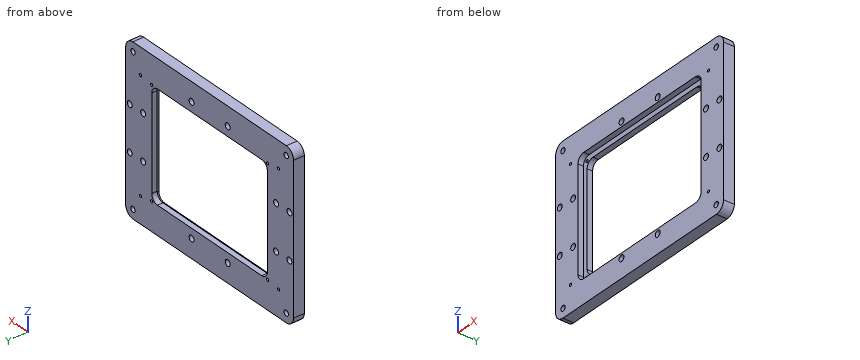
```python
from build123d import *

# Parameters (mm, degrees)
SKETCH_2_W               = 220
SKETCH_2_H               = 150
SKETCH_2_W_2             = 160
SKETCH_2_H_2             = 120
EXTRUDE_1_DEPTH          = 12
SKETCH_3_W               = 170.5
SKETCH_3_H               = 130.5
CUT_EXTRUDE_1_DEPTH      = 6
FILLET_1_R               = 8
FILLET_2_R               = 8
FILLET_3_R               = 8
CUT_EXTRUDE_2_DEPTH      = 134.270401815
CUT_EXTRUDE_2_DEPTH_BACK = 140.270401815
CUT_EXTRUDE_2_START      = 6
SKETCH_4_R               = 1.5
SKETCH_6_W               = 241.523327546
SKETCH_6_H               = 183.41982478
SKETCH_6_W_2             = 210.674446864
SKETCH_6_H_2             = 143.430858526
EXTRUDE_2_DEPTH          = 12
SKETCH_5_R               = 3.3655
CUT_EXTRUDE_3_DEPTH      = 22
SKETCH_7_R               = 3
CUT_EXTRUDE_4_DEPTH      = 22
FILLET_4_R               = 6
FILLET_5_R               = 6
FILLET_6_R               = 6
FILLET_7_R               = 6
SKETCH_14_W              = 180
SKETCH_14_H              = 7.031256172
SKETCH_14_R              = 2
EXTRUDE_3_DEPTH          = 12
SKETCH_14_W_2            = 130
SKETCH_14_H_2            = 7
EXTRUDE_3_2_DEPTH        = 12
EXTRUDE_3_3_DEPTH        = 12
EXTRUDE_3_4_DEPTH        = 12
SKETCH_15_W              = 460.716543434
SKETCH_15_H              = 403.643057854
SKETCH_15_W_2            = 232.32954725
SKETCH_15_H_2            = 183.087092282
CUT_EXTRUDE_8_DEPTH      = 105
FILLET_8_R               = 10


with BuildPart() as part:
    # Эскиз2 → Бобышка-Вытянуть1 (new body)
    with BuildSketch(Plane(origin=(0, 0, 0), x_dir=(1, 0, 0), z_dir=(0, 1, 0))):
        Rectangle(SKETCH_2_W, SKETCH_2_H)
        Rectangle(SKETCH_2_W_2, SKETCH_2_H_2, mode=Mode.SUBTRACT)
    extrude(amount=EXTRUDE_1_DEPTH)

    # Эскиз3 → Вырез-Вытянуть1 (cut)
    with BuildSketch(Plane.XZ):
        Rectangle(SKETCH_3_W, SKETCH_3_H)
    extrude(amount=-CUT_EXTRUDE_1_DEPTH, mode=Mode.SUBTRACT)

    # Скругление1
    fillet_1_edges = [part.edges().sort_by_distance(p)[0] for p in [
        (80, 9, 60),
    ]]
    fillet(fillet_1_edges, radius=FILLET_1_R)

    # Скругление2
    fillet_2_edges = [part.edges().sort_by_distance(p)[0] for p in [
        (85.25, 3, 65.25),
    ]]
    fillet(fillet_2_edges, radius=FILLET_2_R)

    # Скругление3
    fillet_3_edges = [part.edges().sort_by_distance(p)[0] for p in [
        (80, 9, -60),
        (-80, 9, -60),
        (-80, 9, 60),
        (85.25, 3, -65.25),
        (-85.25, 3, -65.25),
        (-85.25, 3, 65.25),
    ]]
    fillet(fillet_3_edges, radius=FILLET_3_R)

    # Эскиз4 → Вырез-Вытянуть2 (cut, two sides: drawn at the far end of the back side and taken through both)
    with BuildSketch(Plane.XZ.offset(-6).offset(CUT_EXTRUDE_2_START - CUT_EXTRUDE_2_DEPTH_BACK)):
        with Locations(Location((-80.15, 60.15, 0), (0, 0, 270))):
            Circle(SKETCH_4_R)
        with Locations(Location((-80.15, -60.15, 0), (0, 0, 270))):
            Circle(SKETCH_4_R)
        with Locations(Location((80.15, -60.15, 0), (0, 0, 270))):
            Circle(SKETCH_4_R)
        with Locations(Location((80.15, 60.15, 0), (0, 0, 270))):
            Circle(SKETCH_4_R)
        with Locations(Location((-95.5, 62.5, 0), (0, 0, 270))):
            Circle(SKETCH_4_R)
        with Locations(Location((-95.5, -62.5, 0), (0, 0, 270))):
            Circle(SKETCH_4_R)
        with Locations(Location((95.5, -62.5, 0), (0, 0, 270))):
            Circle(SKETCH_4_R)
        with Locations(Location((95.5, 62.5, 0), (0, 0, 270))):
            Circle(SKETCH_4_R)
    extrude(amount=CUT_EXTRUDE_2_DEPTH + CUT_EXTRUDE_2_DEPTH_BACK, mode=Mode.SUBTRACT)

    # Эскиз6 → Бобышка-Вытянуть2 (add)
    with BuildSketch(Plane.XZ):
        Rectangle(SKETCH_6_W, SKETCH_6_H)
        Rectangle(SKETCH_6_W_2, SKETCH_6_H_2, mode=Mode.SUBTRACT)
    extrude(amount=-EXTRUDE_2_DEPTH)

    # Эскиз5 → Вырез-Вытянуть3 (cut)
    with BuildSketch(Plane.XZ):
        with Locations(Location((-92.006407499, -25, 0), (0, 0, 270))):
            Circle(SKETCH_5_R)
        with Locations(Location((-110.497607499, -25, 0), (0, 0, 270))):
            Circle(SKETCH_5_R)
        with Locations(Location((-110.497607499, 25.000000038, 0), (0, 0, 270))):
            Circle(SKETCH_5_R)
        with Locations(Location((-92.006407499, 25.000000038, 0), (0, 0, 270))):
            Circle(SKETCH_5_R)
        with Locations(Location((92.006407499, 25.000000038, 0), (0, 0, 270))):
            Circle(SKETCH_5_R)
        with Locations(Location((110.497607499, 25.000000038, 0), (0, 0, 270))):
            Circle(SKETCH_5_R)
        with Locations(Location((110.497607499, -25, 0), (0, 0, 270))):
            Circle(SKETCH_5_R)
        with Locations(Location((92.006407499, -25, 0), (0, 0, 270))):
            Circle(SKETCH_5_R)
        with Locations(Location((25, 70.661122045, 0), (0, 0, 270))):
            Circle(SKETCH_5_R)
        with Locations(Location((-25.000000038, 70.661122045, 0), (0, 0, 270))):
            Circle(SKETCH_5_R)
        with Locations(Location((-25.000000038, -70.661122045, 0), (0, 0, 270))):
            Circle(SKETCH_5_R)
        with Locations(Location((25, -70.661122045, 0), (0, 0, 270))):
            Circle(SKETCH_5_R)
    extrude(amount=-CUT_EXTRUDE_3_DEPTH, mode=Mode.SUBTRACT)

    # Эскиз7 → Вырез-Вытянуть4 (cut)
    with BuildSketch(Plane.XZ):
        with Locations(Location((-106.020205838, -81.450824183, 0), (0, 0, 270))):
            Circle(SKETCH_7_R)
        with Locations(Location((-106.020205838, 81.450824183, 0), (0, 0, 270))):
            Circle(SKETCH_7_R)
        with Locations(Location((106.020205838, 81.450824183, 0), (0, 0, 270))):
            Circle(SKETCH_7_R)
        with Locations(Location((106.020205838, -81.450824183, 0), (0, 0, 270))):
            Circle(SKETCH_7_R)
    extrude(amount=-CUT_EXTRUDE_4_DEPTH, mode=Mode.SUBTRACT)

    # Скругление4
    fillet_4_edges = [part.edges().sort_by_distance(p)[0] for p in [
        (120.761663773, 6, 91.70991239),
    ]]
    fillet(fillet_4_edges, radius=FILLET_4_R)

    # Скругление5
    fillet_5_edges = [part.edges().sort_by_distance(p)[0] for p in [
        (120.761663773, 6, -91.70991239),
    ]]
    fillet(fillet_5_edges, radius=FILLET_5_R)

    # Скругление6
    fillet_6_edges = [part.edges().sort_by_distance(p)[0] for p in [
        (-120.761663773, 6, -91.70991239),
    ]]
    fillet(fillet_6_edges, radius=FILLET_6_R)

    # Скругление7
    fillet_7_edges = [part.edges().sort_by_distance(p)[0] for p in [
        (-120.761663773, 6, 91.70991239),
    ]]
    fillet(fillet_7_edges, radius=FILLET_7_R)


with BuildPart() as body_2:
    # Эскиз14 → Бобышка-Вытянуть3 (new body)
    with BuildSketch(Plane(origin=(0, 12, 0), x_dir=(1, 0, 0), z_dir=(0, 1, 0))):
        with Locations((1.41446019, 109.44602362)):
            Rectangle(SKETCH_14_W, SKETCH_14_H)
        with Locations(Location((-81.58561634, 109.413291168, 0), (0, 0, 270))):
            Circle(SKETCH_14_R, mode=Mode.SUBTRACT)
        with Locations(Location((1.41446019, 109.413291168, 0), (0, 0, 270))):
            Circle(SKETCH_14_R, mode=Mode.SUBTRACT)
        with Locations(Location((84.41453672, 109.413291168, 0), (0, 0, 270))):
            Circle(SKETCH_14_R, mode=Mode.SUBTRACT)
    extrude(amount=-EXTRUDE_3_DEPTH)


with BuildPart() as body_3:
    # Эскиз14 → Extrude 3 2 (new body)
    with BuildSketch(Plane(origin=(0, 12, 0), x_dir=(1, 0, 0), z_dir=(0, 1, 0))):
        with Locations((-6.451217143, 118.582116541)):
            Rectangle(SKETCH_14_W_2, SKETCH_14_H_2)
        with Locations(Location((51.548782857, 118.582116541, 0), (0, 0, 270))):
            Circle(SKETCH_14_R, mode=Mode.SUBTRACT)
        with Locations(Location((-6.451217143, 118.582116541, 0), (0, 0, 270))):
            Circle(SKETCH_14_R, mode=Mode.SUBTRACT)
        with Locations(Location((-64.451217143, 118.582116541, 0), (0, 0, 270))):
            Circle(SKETCH_14_R, mode=Mode.SUBTRACT)
    extrude(amount=-EXTRUDE_3_2_DEPTH)


with BuildPart() as body_4:
    # Эскиз14 → Extrude 3 3 (new body)
    with BuildSketch(Plane(origin=(0, 12, 0), x_dir=(1, 0, 0), z_dir=(0, 1, 0))):
        with Locations((1.538593971, 129.106977772)):
            Rectangle(SKETCH_14_W, SKETCH_14_H)
        with Locations(Location((-81.461482559, 129.07424532, 0), (0, 0, 270))):
            Circle(SKETCH_14_R, mode=Mode.SUBTRACT)
        with Locations(Location((1.538593971, 129.07424532, 0), (0, 0, 270))):
            Circle(SKETCH_14_R, mode=Mode.SUBTRACT)
        with Locations(Location((84.538670501, 129.07424532, 0), (0, 0, 270))):
            Circle(SKETCH_14_R, mode=Mode.SUBTRACT)
    extrude(amount=-EXTRUDE_3_3_DEPTH)


with BuildPart() as body_5:
    # Эскиз14 → Extrude 3 4 (new body)
    with BuildSketch(Plane(origin=(0, 12, 0), x_dir=(1, 0, 0), z_dir=(0, 1, 0))):
        with Locations((-6.327083362, 138.243070693)):
            Rectangle(SKETCH_14_W_2, SKETCH_14_H_2)
        with Locations(Location((51.672916638, 138.243070693, 0), (0, 0, 270))):
            Circle(SKETCH_14_R, mode=Mode.SUBTRACT)
        with Locations(Location((-6.327083362, 138.243070693, 0), (0, 0, 270))):
            Circle(SKETCH_14_R, mode=Mode.SUBTRACT)
        with Locations(Location((-64.327083362, 138.243070693, 0), (0, 0, 270))):
            Circle(SKETCH_14_R, mode=Mode.SUBTRACT)
    extrude(amount=-EXTRUDE_3_4_DEPTH)


with BuildPart() as cut_extrude_8_tool:
    # Эскиз15 → Вырез-Вытянуть8 (new body)
    with BuildSketch(Plane.XZ):
        Rectangle(SKETCH_15_W, SKETCH_15_H)
        Rectangle(SKETCH_15_W_2, SKETCH_15_H_2, mode=Mode.SUBTRACT)
    extrude(amount=-CUT_EXTRUDE_8_DEPTH)


with BuildPart() as part_1:
    add(part.part)

    # Вырез-Вытянуть8: cut by cut_extrude_8_tool
    add(cut_extrude_8_tool.part, mode=Mode.SUBTRACT)

    # Скругление8
    fillet_8_edges = [part_1.edges().sort_by_distance(p)[0] for p in [
        (116.164773625, 6, -91.543546141),
        (-116.164773625, 6, -91.543546141),
        (-116.164773625, 6, 91.543546141),
        (116.164773625, 6, 91.543546141),
    ]]
    fillet(fillet_8_edges, radius=FILLET_8_R)


with BuildPart() as body_2_1:
    add(body_2.part)

    # Вырез-Вытянуть8: cut by cut_extrude_8_tool
    add(cut_extrude_8_tool.part, mode=Mode.SUBTRACT)


with BuildPart() as body_3_1:
    add(body_3.part)

    # Вырез-Вытянуть8: cut by cut_extrude_8_tool
    add(cut_extrude_8_tool.part, mode=Mode.SUBTRACT)


with BuildPart() as body_4_1:
    add(body_4.part)

    # Вырез-Вытянуть8: cut by cut_extrude_8_tool
    add(cut_extrude_8_tool.part, mode=Mode.SUBTRACT)


with BuildPart() as body_5_1:
    add(body_5.part)

    # Вырез-Вытянуть8: cut by cut_extrude_8_tool
    add(cut_extrude_8_tool.part, mode=Mode.SUBTRACT)


solid = part_1.part
```
The listing builds one solid part. Answer for the finished solid, in the listing's coordinates (mm). Give positions to 0.01 mm unless a question says otherwise; leave off trailing zeros. Write each loop counter-clockwise with the first axis right and the second up, starting at its lowest first coordinate (ties: lowest second). Pieces come first, ordered by that corner, then holes. Notation, with made-up numbers: (64, 33) - (69, 33) arc R12 cw to (69, 51) - close; hole circle Ø9 at (6.25, 9). An arc over 180 degrees is marked (long way). Use one line per item in the form item = value. Start each with the question number.
1) Find section B-B on z = 25. Determine the outline of the cut face in (x, y), plus the area to 3 significant figures.
2) Find section C-C on z = 71. Determine the outline of the cut face in (x, y).
3) Find section D-D on y = 3.5. Count the separate pieces of the cut face and the enclosed holes in it, plus the area to 3 significant figures.
4) Find section A-A on x = 25. Determine the outline of the cut face in (y, z).
5) A flat-ended cylindrical pin translates along its axis: pin 1 Ø4 at (x, z) = (-92.01, -25) entering from -Y. Find the tip coordinate at first contact, or state that the pin passes through.
6) Consider line 1 along Z through (x, y) = (25.5, 3.75); line 2 along X through (y, z) = (8.7, -60.15); line 3 along Z through (x, y) = (-54, 11.25). Determine where each line is inside the solid, lowest interval first. Write a range as from..to.
Geometry results:
q1.outline = (-116.16, 0) - (-113.86, 0) - (-113.86, 12) - (-116.16, 12) - close; (-107.13, 0) - (-95.37, 0) - (-95.37, 12) - (-107.13, 12) - close; (-88.64, 0) - (-85.25, 0) - (-85.25, 6) - (-80, 6) - (-80, 12) - (-88.64, 12) - close; (80, 6) - (85.25, 6) - (85.25, 0) - (88.64, 0) - (88.64, 12) - (80, 12) - close; (95.37, 0) - (107.13, 0) - (107.13, 12) - (95.37, 12) - close; (113.86, 0) - (116.16, 0) - (116.16, 12) - (113.86, 12) - close
q1.area = 482 mm2
q2.outline = (-116.16, 0) - (-28.35, 0) - (-28.35, 12) - (-116.16, 12) - close; (-21.65, 0) - (21.65, 0) - (21.65, 12) - (-21.65, 12) - close; (28.35, 0) - (116.16, 0) - (116.16, 12) - (28.35, 12) - close
q3.separate_pieces = 1
q3.enclosed_holes = 21
q3.area = 19,700 mm2
q4.outline = (0, -91.54) - (12, -91.54) - (12, -74.03) - (0, -74.03) - close; (0, -67.3) - (12, -67.3) - (12, -60) - (6, -60) - (6, -65.25) - (0, -65.25) - close; (0, 65.25) - (6, 65.25) - (6, 60) - (12, 60) - (12, 67.3) - (0, 67.3) - close; (0, 74.03) - (12, 74.03) - (12, 91.54) - (0, 91.54) - close
q5.pin_1 = through
q6.line_1 = -91.54..-73.99, -67.33..-65.25, 65.25..67.33, 73.99..91.54
q6.line_2 = -116.16..-81.65, -78.65..78.65, 81.65..116.16
q6.line_3 = -91.54..-60, 60..91.54
